from build123d import *

# Parameters (mm, degrees)
CROQUIS1_W                   = 482.6
CROQUIS1_H                   = 157.988
BRIDA_BASE1_DEPTH            = 1.524
CROQUIS6_R                   = 3.9624
CROQUIS6_W                   = 6.35
CROQUIS6_H                   = 3.048
CORTAR_EXTRUIR1_DEPTH        = 254.905621466
BRIDA_START                  = -218.948
BRIDA_DE_ARISTA1_DEPTH       = 437.896
BRIDA_START_2                = -219.1004
BRIDA_DE_ARISTA1_2_OUTLINE_W = 0.1524
BRIDA_DE_ARISTA1_2_OUTLINE_H = 1.524
BRIDA_DE_ARISTA1_2_DEPTH     = 0.1524
BRIDA_START_3                = 218.948
BRIDA_DE_ARISTA1_3_OUTLINE_W = 0.1524
BRIDA_DE_ARISTA1_3_OUTLINE_H = 1.524
BRIDA_DE_ARISTA1_3_DEPTH     = 0.1524
BRIDA_DE_ARISTA1_4_DEPTH     = 437.896
CROQUIS13_R                  = 2.794
CROQUIS13_R_2                = 1.2065
CROQUIS13_R_3                = 3.937
CROQUIS13_W                  = 124.714
CROQUIS13_H                  = 139.7
CORTAR_EXTRUIR2_DEPTH        = 27.178


# Read off the part's stored shape, not the designer's step: Brida de arista1
# Sheet-metal steps are written as plain solids
with BuildPart() as part:
    # Croquis1 → Brida base1 (new body)
    with BuildSketch(Plane.XY):
        Rectangle(CROQUIS1_W, CROQUIS1_H)
    extrude(amount=-BRIDA_BASE1_DEPTH)

    # Croquis6 → Cortar-Extruir1 (cut, through all)
    with BuildSketch(Plane.XY):
        with Locations((231.648, 79.502)):
            Circle(CROQUIS6_R)
        with Locations((-231.648, 79.502)):
            Circle(CROQUIS6_R)
        with Locations((-231.648, -79.502)):
            Circle(CROQUIS6_R)
        with Locations((231.648, -79.502)):
            Circle(CROQUIS6_R)
        with Locations((-222.123, 77.47)):
            Rectangle(CROQUIS6_W, CROQUIS6_H)
        with Locations((222.123, 77.47)):
            Rectangle(CROQUIS6_W, CROQUIS6_H)
        with Locations((-222.123, -77.47)):
            Rectangle(CROQUIS6_W, CROQUIS6_H)
        with Locations((222.123, -77.47)):
            Rectangle(CROQUIS6_W, CROQUIS6_H)
    extrude(amount=-CORTAR_EXTRUIR1_DEPTH, mode=Mode.SUBTRACT)

    # Brida de arista1 outline → Brida de arista1 (cut)
    with BuildSketch(Plane.YZ.offset(BRIDA_START)):
        with BuildLine():
            ThreePointArc((-78.585645431, -1.524), (-77.47, -0.408354569), (-75.946, 0))
            Line((-75.946, 0), (-78.994, 0))
            Line((-78.994, 0), (-78.994, -1.524))
            Line((-78.994, -1.524), (-78.585645431, -1.524))
        make_face()
        with BuildLine():
            Line((78.994, 0), (75.946, 0))
            ThreePointArc((75.946, 0), (77.47, -0.408354569), (78.585645431, -1.524))
            Line((78.585645431, -1.524), (78.994, -1.524))
            Line((78.994, -1.524), (78.994, 0))
        make_face()
    extrude(amount=BRIDA_DE_ARISTA1_DEPTH, mode=Mode.SUBTRACT)

    # Brida de arista1 2 outline → Brida de arista1 2 (cut)
    with BuildSketch(Plane.YZ.offset(BRIDA_START_2)):
        with Locations((-75.8698, -0.762)):
            Rectangle(BRIDA_DE_ARISTA1_2_OUTLINE_W, BRIDA_DE_ARISTA1_2_OUTLINE_H)
        with Locations((75.8698, -0.762)):
            Rectangle(BRIDA_DE_ARISTA1_2_OUTLINE_W, BRIDA_DE_ARISTA1_2_OUTLINE_H)
    extrude(amount=BRIDA_DE_ARISTA1_2_DEPTH, mode=Mode.SUBTRACT)

    # Brida de arista1 3 outline → Brida de arista1 3 (cut)
    with BuildSketch(Plane.YZ.offset(BRIDA_START_3)):
        with Locations((-75.8698, -0.762)):
            Rectangle(BRIDA_DE_ARISTA1_3_OUTLINE_W, BRIDA_DE_ARISTA1_3_OUTLINE_H)
        with Locations((75.8698, -0.762)):
            Rectangle(BRIDA_DE_ARISTA1_3_OUTLINE_W, BRIDA_DE_ARISTA1_3_OUTLINE_H)
    extrude(amount=BRIDA_DE_ARISTA1_3_DEPTH, mode=Mode.SUBTRACT)

    # Brida de arista1 4 outline → Brida de arista1 4 (add)
    with BuildSketch(Plane.YZ.offset(BRIDA_START)):
        with BuildLine():
            ThreePointArc((-77.47, -3.048), (-77.023630735, -1.970369265), (-75.946, -1.524))
            Line((-75.946, -1.524), (-78.585645431, -1.524))
            ThreePointArc((-78.585645431, -1.524), (-78.890141918, -2.259119551), (-78.994, -3.048))
            Line((-78.994, -3.048), (-78.994, -16.002))
            Line((-78.994, -16.002), (-77.47, -16.002))
            Line((-77.47, -16.002), (-77.47, -3.048))
        make_face()
        with BuildLine():
            Line((78.585645431, -1.524), (75.946, -1.524))
            ThreePointArc((75.946, -1.524), (77.023630735, -1.970369265), (77.47, -3.048))
            Line((77.47, -3.048), (77.47, -16.002))
            Line((77.47, -16.002), (78.994, -16.002))
            Line((78.994, -16.002), (78.994, -3.048))
            ThreePointArc((78.994, -3.048), (78.890141918, -2.259119551), (78.585645431, -1.524))
        make_face()
    extrude(amount=BRIDA_DE_ARISTA1_4_DEPTH)

    # Croquis13 → Cortar-Extruir2 (cut)
    with BuildSketch(Plane.XY):
        with Locations((-106.68, 14.478)):
            Circle(CROQUIS13_R)
        with Locations((-106.68, -14.224)):
            Circle(CROQUIS13_R)
        with Locations((-107.95, 46.99)):
            Circle(CROQUIS13_R_2)
        with Locations((-171.45, 46.99)):
            Circle(CROQUIS13_R_2)
        with Locations((-231.648, -3.302)):
            Circle(CROQUIS13_R_3)
        with Locations((11.557, 0)):
            Rectangle(CROQUIS13_W, CROQUIS13_H)
    extrude(amount=-CORTAR_EXTRUIR2_DEPTH, mode=Mode.SUBTRACT)


solid = part.part
Model file for the job. Use its own axes, mm. A direction names the side the tool comes from. Give positions to 0.01 mm unless a question says otherwise; leave off trailing zeros. Order: outer loops, then holes, each group sorted by start corner. A loop starts at its lowest first (then second) coordinate and runs counter-clockwise, first axis right, second up. Notation, with made-up numbers: (81.25, 32) - (88.25, 32) arc R12 ccw to (88.25, 54) - close; hole circle Ø8 at (36, 47.25). An arc over 180 degrees is marked (long way). Return JSON: item names as keys, results as strings.
1) Cut at B-B, the plane y = -47.5. Give the cut face in (x, z).
Geometry says:
{"outline": "(-241.3, -1.52) - (-50.8, -1.52) - (-50.8, 0) - (-241.3, 0) - close; (73.91, -1.52) - (241.3, -1.52) - (241.3, 0) - (73.91, 0) - close"}
2) Cut at D-D, the plane x = 167. Give the cut face in (y, z).
Geometry says:
{"outline": "(-78.99, -16) - (-77.47, -16) - (-77.47, -3.05) arc R1.52 cw to (-75.95, -1.52) - (75.95, -1.52) arc R1.52 cw to (77.47, -3.05) - (77.47, -16) - (78.99, -16) - (78.99, -3.05) arc R3.05 ccw to (75.95, 0) - (-75.95, 0) arc R3.05 ccw to (-78.99, -3.05) - close"}
3) Cut at A-A, the plane x = 20. Give the cut face in (y, z).
Geometry says:
{"outline": "(-78.99, -16) - (-77.47, -16) - (-77.47, -3.05) arc R1.52 cw to (-75.95, -1.52) - (-69.85, -1.52) - (-69.85, 0) - (-75.95, 0) arc R3.05 ccw to (-78.99, -3.05) - close; (69.85, -1.52) - (75.95, -1.52) arc R1.52 cw to (77.47, -3.05) - (77.47, -16) - (78.99, -16) - (78.99, -3.05) arc R3.05 ccw to (75.95, 0) - (69.85, 0) - close"}
4) Probe line 1 (Y direction, x = -4, z = -2.5); line 2 (Y direction, x = -107.95, z = -0.35); line 3 (Y direction, x = 111.5, z = -8). List the from-to ranges inside material, lowest first. Write a range as from..to.
Geometry says:
{"line 1": "-78.94..-77.37, 77.37..78.94", "line 2": "-77.36..-16.71, -11.74..11.99, 16.97..45.78, 48.2..77.36", "line 3": "-78.99..-77.47, 77.47..78.99"}
5) 3-axis set-ups, long thin cutter, end or side, ignore diameter. For faces 1 (the flat face through (-3, 77.47, -9)), 2 (the flat face through (-3, -78.994, -9)): which of +Z, -Z, +X, -X, +Y, -Y reach the whole face in a straight line?
Geometry says:
{"face 1": "-Z, +X, -X", "face 2": "+Z, -Z, +X, -X, -Y"}
6) Cut at C-C, the plane z = -12.5. Give the cut face in (x, y), plus the area to 3 significant figures.
Geometry says:
{"outline": "(-218.95, -78.99) - (218.95, -78.99) - (218.95, -77.47) - (-218.95, -77.47) - close; (-218.95, 77.47) - (218.95, 77.47) - (218.95, 78.99) - (-218.95, 78.99) - close", "area": "1,330 mm²"}
7) Pull direction Y, two halves, no side cores. Call faces 3 (the flat face through (-3, 78.994, -10)), 4 (the flat face through (-57, 1, 0)), 5 (the cylindrical face through (-227.9, -2.1, -0.8)): pulls with the +Y half, pulls with the -Y half, needs draft (parallel to the pull), parting line crosses it, or undercut.
Geometry says:
{"face 3": "pulls with the +Y half", "face 4": "needs draft", "face 5": "undercut"}
8) Flat gauge pins, fed straight in: P1, Ø5, axis at y = -27.5, z = -6.5, coming from the -X side; P2, Ø3, axis at x = -107.95, y = 46.99, coming from the -Z side; P3, Ø3.5, axis at y = 76.5, z = -7.5, coming from the -X side; P4, Ø0.8, axis at x = -16.5, z = -1, coming from the +Y side. Where does each tip first touch, or does it go through?
Geometry says:
{"P1": "through", "P2": "z = -1.52", "P3": "x = -218.95", "P4": "y = 78.51"}
